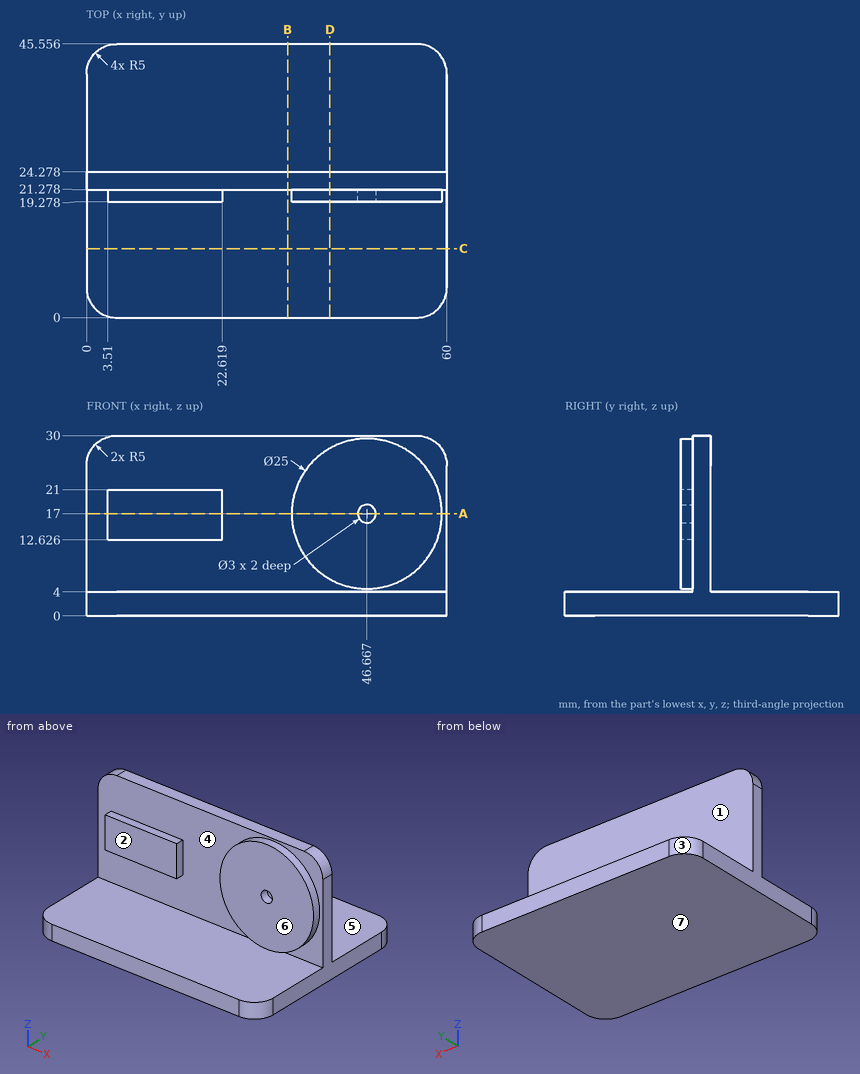
Part print with two shaded views. Sizes in mm from the minimum x, y, z corner. A direction names the side the tool comes from. Give positions to 0.01 mm unless a question says otherwise; leave off trailing zeros. Loops run counter-clockwise (first coordinate to the right, second up) from the corner with the lowest first, then second, coordinate; pieces in that order, holes last. Notation, with made-up numbers: (6, -5) -> (55, -5) arc R33 ccw to (55, 34) -> close; hole circle Ø8 at (74.25, 22). An arc over 180 degrees is marked (long way). One line per question, with ' | ' between items.
Q1. Cut at A-A, the plane z = 17. Write the cut outline in (x, y).
Filled sheet:
outline: (0, 21.28) -> (3.51, 21.28) -> (3.51, 19.28) -> (22.62, 19.28) -> (22.62, 21.28) -> (34.17, 21.28) -> (34.17, 19.28) -> (45.17, 19.28) -> (45.17, 21.28) -> (48.17, 21.28) -> (48.17, 19.28) -> (59.17, 19.28) -> (59.17, 21.28) -> (60, 21.28) -> (60, 24.28) -> (0, 24.28) -> close
Q2. Drop flat-ended pins along their axis: pin 1 (1.8 mm diameter, centred on x = 46.67, z = 17, fed in from +Y); pin 2 (2 mm diameter, centred on x = 38.5, y = 31.5, fed in from -Z); pin 3 (0.6 mm diameter, centred on y = 20, z = 15.5, fed in from -X); pin 4 (1.6 mm diameter, centred on x = 17, y = 20, fed in from +Z). Give the stop position or say it passes through.
Filled sheet:
pin 1: stops at y = 24.28 | pin 2: stops at z = 0 | pin 3: stops at x = 3.51 | pin 4: stops at z = 21
Q3. Drill centre lines: line 1 along Y through (x, z) = (51.5, 18); line 2 along Z through (x, y) = (19, 30); line 3 along Y through (x, z) = (17.5, 27). Where is each one in solid material? Low to high. Write a range as [from, to].
Filled sheet:
line 1: y = [19.28, 24.28] | line 2: z = [0, 4] | line 3: y = [21.28, 24.28]
Q4. Pull direction Z, two halves, no side cores. Call the marked faces 4, 5, 6 and 7: pulls with the +Z half, pulls with the -Z half, needs draft (parallel to the pull), parting line crosses it, or undercut.
Filled sheet:
face 4: undercut | face 5: pulls with the +Z half | face 6: needs draft | face 7: pulls with the -Z half
Q5. Cut at D-D, the plane x = 40.5. Write the cut outline in (y, z) (1 decimal).
Filled sheet:
outline: (0, 0) -> (45.6, 0) -> (45.6, 4) -> (24.3, 4) -> (24.3, 30) -> (21.3, 30) -> (21.3, 27.9) -> (19.3, 27.9) -> (19.3, 6.1) -> (21.3, 6.1) -> (21.3, 4) -> (0, 4) -> close
Q6. Tool access for the marked faces 1, 2 and 3: list every direction of +Z, -Z, +X, -X, +Y, -Y with a clear straight run to the whole face (end or side of a thin tool).
Filled sheet:
face 1: +Z, +X, -X, +Y | face 2: +Z, +X, -X, -Y | face 3: +Z, -Z, -X, +Y
Q7. Cut at B-B, the plane x = 33.5. Write the cut outline in (y, z) (1 decimal).
Filled sheet:
outline: (0, 0) -> (45.6, 0) -> (45.6, 4) -> (24.3, 4) -> (24.3, 30) -> (21.3, 30) -> (21.3, 4) -> (0, 4) -> close
Q8. Cut at C-C, the plane y = 11.5. Write the cut outline in (x, z), plus the area to 3 significant figures.
Filled sheet:
outline: (0, 0) -> (60, 0) -> (60, 4) -> (0, 4) -> close | area: 240 mm²
